```python
from build123d import *

# Parameters (mm, degrees)
SKETCH1_W           = 40
SKETCH1_H           = 16.8
BOSS_EXTRUDE1_DEPTH = 28
FILLET2_R           = 10
SKETCH3_W           = 9.871170143
SKETCH3_H           = 10
SKETCH3_W_2         = 30
BOSS_EXTRUDE2_DEPTH = 16.8
SKETCH2_R           = 3
SKETCH2_R_2         = 1.25
CUT_EXTRUDE1_DEPTH  = 16.8
SKETCH4_R           = 1.25
CUT_EXTRUDE2_DEPTH  = 36.419768492


with BuildPart() as part:
    # Sketch1 → Boss-Extrude1 (new body)
    with BuildSketch(Plane(origin=(0, 0, 0), x_dir=(1, 0, 0), z_dir=(0, 1, 0))):
        Rectangle(SKETCH1_W, SKETCH1_H)
    extrude(amount=BOSS_EXTRUDE1_DEPTH)

    # Fillet2
    # the kernel refuses this fillet: 10 mm, written as the material it takes off along each edge
    with BuildSketch(Plane(origin=(20, -25, -8.4), x_dir=(0, 0, 1), z_dir=(0, 1, 0)), Plane(origin=(20, -25, 8.4), x_dir=(-1, 0, 0), z_dir=(0, 1, 0))) as fillet2_piece_1:
        with BuildLine():
            CenterArc((FILLET2_R, -FILLET2_R), FILLET2_R, 90, 90)
            Line((0, -FILLET2_R), (0, 0))
            Line((0, 0), (FILLET2_R, 0))
        make_face()
    extrude(amount=78, mode=Mode.SUBTRACT)

    # Sketch3 → Boss-Extrude2 (add)
    with BuildSketch(Plane.XY.offset(8.4)):
        with Locations((14.935585072, 9)):
            Rectangle(SKETCH3_W, SKETCH3_H)
        with Locations((14.935585072, 19)):
            Rectangle(SKETCH3_W, SKETCH3_H)
        with Locations((-5, 19)):
            Rectangle(SKETCH3_W_2, SKETCH3_H)
        with Locations((-5, 9)):
            Rectangle(SKETCH3_W_2, SKETCH3_H)
    extrude(amount=-BOSS_EXTRUDE2_DEPTH)

    # Sketch2 → Cut-Extrude1 (cut)
    with BuildSketch(Plane.XY.offset(8.4)):
        with Locations((-14.25, 14)):
            Circle(SKETCH2_R)
        with Locations((9.5, 14)):
            Circle(SKETCH2_R_2)
        with Locations((0.25, 20.75)):
            Circle(SKETCH2_R_2)
        with Locations((0.25, 7.25)):
            Circle(SKETCH2_R_2)
    extrude(amount=-CUT_EXTRUDE1_DEPTH, mode=Mode.SUBTRACT)

    # Sketch4 → Cut-Extrude2 (cut, through all)
    with BuildSketch(Plane(origin=(0, 28, 0), x_dir=(1, 0, 0), z_dir=(0, 1, 0))):
        with Locations(Location((-11, 0, 0), (0, 0, 270))):
            Circle(SKETCH4_R)
        with Locations(Location((1, 0, 0), (0, 0, 270))):
            Circle(SKETCH4_R)
        with Locations(Location((13, 0, 0), (0, 0, 270))):
            Circle(SKETCH4_R)
    extrude(amount=-CUT_EXTRUDE2_DEPTH, mode=Mode.SUBTRACT)


solid = part.part
```
Input: part model. Units: mm. Frame: model coordinates. A direction names the side the tool comes from. Give positions to 0.01 mm unless a question says otherwise; leave off trailing zeros. Order: outer loops, then holes, each group sorted by start corner. A loop starts at its lowest first (then second) coordinate and runs counter-clockwise, first axis right, second up. Notation, with made-up numbers: (87.5, 1.25) - (144.5, 1.25) arc R18 cw to (144.5, 9.25) - close; hole circle Ø8 at (54.25, -17.75). An arc over 180 degrees is marked (long way). Put each result on its own line as item: value.
Item 1: Access query for faces 5 (the flat face through (17, 4, 6)), 6 (the flat face through (18, 24, -6)), 7 (the cylindrical face through (16.56, 1.97, -5.95)). Directions: +Z, -Z, +X, -X, +Y, -Y. A direction counts if a zero-diameter tool reaches every point of the face in a straight line with its end or side. Return the directions, or none.
Found:
face 5: +Z, +X, -Y
face 6: -Z, +X, +Y
face 7: -Z, +X, -Y
Item 2: Draft query along Y for faces 1 (the cylindrical face through (-17.247, 14.132, 0.118)), 2 (the cylindrical face through (16.56, 25.97, -5.95)), 3 (the cylindrical face through (-1, 20.8, 0.1)), 4 (the flat face through (0, 28, -2)). Return one class per face: +Y half, -Y half, draft (parallel to the pull), parting line (faces both ways), or undercut.
Found:
face 1: undercut
face 2: draft
face 3: undercut
face 4: +Y half
Item 3: Section query B-B, the plane x = 1. Return loops of the section in (y, z).
Found:
outline: (0, -8.4) - (6.25, -8.4) - (6.25, -1.25) - (0, -1.25) - close; (0, 1.25) - (6.25, 1.25) - (6.25, 8.4) - (0, 8.4) - close; (8.25, -8.4) - (19.75, -8.4) - (19.75, -1.25) - (8.25, -1.25) - close; (8.25, 1.25) - (19.75, 1.25) - (19.75, 8.4) - (8.25, 8.4) - close; (21.75, -8.4) - (28, -8.4) - (28, -1.25) - (21.75, -1.25) - close; (21.75, 1.25) - (28, 1.25) - (28, 8.4) - (21.75, 8.4) - close
Item 4: Section query A-A, the plane y = 20.75. Return loops of the section in (x, z).
Found:
outline: (-20, -8.4) - (-1, -8.4) - (-1, 8.4) - (-20, 8.4) - close; (1.5, -8.4) - (19.87, -8.4) - (19.87, 8.4) - (1.5, 8.4) - (1.5, 1.15) arc R1.25 cw to (1.5, -1.15) - close; hole circle Ø2.5 at (-11, 0); hole circle Ø2.5 at (13, 0)
Item 5: Contact query for a flat-ended pin moving along its axis: pin 1 (2 mm diameter, centred on x = 1, z = 0, fed in from -Y). Output: stop coordinate, or through.
Found:
pin 1: passes through
Item 6: Section query C-C, the plane x = -14.25. Return loops of the section in (y, z).
Found:
outline: (0, -8.4) - (11, -8.4) - (11, 8.4) - (0, 8.4) - close; (17, -8.4) - (28, -8.4) - (28, 8.4) - (17, 8.4) - close
Item 7: Section query D-D, the plane z = 2.5. Return loops of the section in (x, y).
Found:
outline: (-20, 0) - (19.12, 0) - (19.12, 4) - (19.87, 4) - (19.87, 24) - (19.12, 24) - (19.12, 28) - (-20, 28) - close; hole circle Ø6 at (-14.25, 14); hole circle Ø2.5 at (0.25, 7.25); hole circle Ø2.5 at (0.25, 20.75); hole circle Ø2.5 at (9.5, 14)
Item 8: Ray query, L1, parallel to Y at x = 0.25, z = 4; L2, parallel to Y at x = -14.25, z = 0.5; L3, parallel to Z at x = 1, y = 13.25. Return the intervals inside material, ascending. Write a range as from..to.
Found:
L1: y = 0..6, 8.5..19.5, 22..28
L2: y = 0..11, 17..28
L3: z = -8.4..-1.25, 1.25..8.4
